```python
from build123d import *

# Parameters (mm, degrees)
SKETCH1_W               = 450
SKETCH1_H               = 170
BOSS_EXTRUDE1_DEPTH     = 6.35
SKETCH2_W               = 15
SKETCH2_H               = 140
CUT_EXTRUDE1_DEPTH      = 1
CUT_EXTRUDE1_DEPTH_BACK = 7.35
FILLET1_R               = 6
FILLET2_R               = 6


with BuildPart() as part:
    # Sketch1 → Boss-Extrude1 (new body)
    with BuildSketch(Plane.XY):
        with Locations((225, 85)):
            Rectangle(SKETCH1_W, SKETCH1_H)
    extrude(amount=BOSS_EXTRUDE1_DEPTH)

    # Sketch2 → Cut-Extrude1 (cut, two sides)
    with BuildSketch(Plane.XY.offset(6.35)) as cut_extrude1_sk:
        with Locations((22.5, 85)):
            Rectangle(SKETCH2_W, SKETCH2_H)
        with Locations((47.5, 85)):
            Rectangle(SKETCH2_W, SKETCH2_H)
        with Locations((72.5, 85)):
            Rectangle(SKETCH2_W, SKETCH2_H)
    extrude(amount=CUT_EXTRUDE1_DEPTH, mode=Mode.SUBTRACT)
    extrude(cut_extrude1_sk.sketch, amount=-CUT_EXTRUDE1_DEPTH_BACK, mode=Mode.SUBTRACT)

    # Fillet1
    fillet1_edges = [part.edges().sort_by_distance(p)[0] for p in [
        (15, 155, 3.175),
        (30, 155, 3.175),
        (40, 155, 3.175),
        (55, 155, 3.175),
        (80, 155, 3.175),
        (65, 155, 3.175),
    ]]
    fillet(fillet1_edges, radius=FILLET1_R)

    # Fillet2
    fillet2_edges = [part.edges().sort_by_distance(p)[0] for p in [
        (30, 15, 3.175),
        (15, 15, 3.175),
        (55, 15, 3.175),
        (40, 15, 3.175),
        (80, 15, 3.175),
        (65, 15, 3.175),
    ]]
    fillet(fillet2_edges, radius=FILLET2_R)


solid = part.part
```
Geometry: final body of the model. Coordinates: model frame, mm. Round coordinates to 2 decimals unless told otherwise and drop trailing zeros. Order: outer loops, then holes, each group sorted by start corner. A loop starts at its lowest first (then second) coordinate and runs counter-clockwise, first axis right, second up. Notation, with made-up numbers: (-26, 62) -> (-11, 62) arc R11 cw to (-11, 80) -> close; hole circle Ø6 at (66.25, 65). An arc over 180 degrees is marked (long way). Use one line per item in the form item = value. Start each with the question number.
1. Cut plane A-A (y = 121). Return the cut outline in (x, z).
2. Line query: probe 1 along X at (y, z) = (102.5, 5.5); probe 2 along Y at (x, z) = (74, 2.5); probe 3 along Y at (x, z) = (79, 5.75). Output: solid intervals per line, ascending.
3. Pin query (flat end, axial travel): pin 1 Ø1.5 at (x, z) = (22.5, 3) entering from -Y. Return the tip coordinate at first contact, or that it passes through.
4. Cut plane B-B (z = 1.75). Return the cut outline in (x, y), then the cut area to 3 significant figures.
Solution:
q1.outline = (0, 0) -> (15, 0) -> (15, 6.35) -> (0, 6.35) -> close; (30, 0) -> (40, 0) -> (40, 6.35) -> (30, 6.35) -> close; (55, 0) -> (65, 0) -> (65, 6.35) -> (55, 6.35) -> close; (80, 0) -> (450, 0) -> (450, 6.35) -> (80, 6.35) -> close
q2.probe_1 = 0 to 15, 30 to 40, 55 to 65, 80 to 450
q2.probe_2 = 0 to 15, 155 to 170
q2.probe_3 = 0 to 17.68, 152.32 to 170
q3.pin_1 = 0
q4.outline = (0, 0) -> (450, 0) -> (450, 170) -> (0, 170) -> close; hole (15, 21) arc R6 ccw to (21, 15) -> (24, 15) arc R6 ccw to (30, 21) -> (30, 149) arc R6 ccw to (24, 155) -> (21, 155) arc R6 ccw to (15, 149) -> close; hole (40, 21) arc R6 ccw to (46, 15) -> (49, 15) arc R6 ccw to (55, 21) -> (55, 149) arc R6 ccw to (49, 155) -> (46, 155) arc R6 ccw to (40, 149) -> close; hole (65, 21) arc R6 ccw to (71, 15) -> (74, 15) arc R6 ccw to (80, 21) -> (80, 149) arc R6 ccw to (74, 155) -> (71, 155) arc R6 ccw to (65, 149) -> close
q4.area = 70,300 mm^2
